Autodesk Inventor part; units mm, degrees
ref_plane "YZ Plane" through (0, 0, 0) normal (1, 0, 0) x (0, 1, 0)
ref_plane "XZ Plane" through (0, 0, 0) normal (0, 1, 0) x (-1, 0, 0)
ref_plane "XY Plane" through (0, 0, 0) normal (0, 0, 1) x (1, 0, 0)
sketch "Sketch1" plane through (0, 0, 0) normal (0, 0, 1) x (1, 0, 0)
  line L0 (-30, 30) -> (30, 30)
  line L1 (30, 30) -> (30, -30)
  line L2 (30, -30) -> (-30, -30)
  line L3 (-30, -30) -> (-30, 30)
  point P0 (0, 0)
  dimension "d0" = 60
  dimension "d1" = 60
  dimension "d2" = 30
  dimension "d3" = 30
extrude "Extrusion1" add sketch "Sketch1" along normal blind 10
sketch "Sketch2" plane through (0, 0, 10) normal (0, 0, 1) x (1, 0, 0)
  line L0 (30, 30) -> (-30, 30)
  line L1 (30, -30) -> (30, 30)
  line L2 (-30, 30) -> (30, 30)
  line L3 (30, 30) -> (30, -5)
  line L4 (30, -5) -> (-30, -5)
  line L5 (-30, -5) -> (-30, 30)
  point P0 (0, 0)
  dimension "d6" = 35
extrude "Extrusion2" add sketch "Sketch2" along normal blind 20
sketch "Sketch3" plane through (0, 0, 10) normal (0, 0, 1) x (1, 0, 0)
  line L0 (-30, -5) -> (30, -5)
  line L1 (-30, -30) -> (30, -30)
  line L2 (-30, -5) -> (30, -5)
  line L3 (30, -5) -> (30, -30)
  line L4 (30, -30) -> (-30, -30)
  line L5 (-30, -30) -> (-30, -5)
  point P0 (0, 0)
extrude "Extrusion3" add sketch "Sketch3" along normal blind 50
sketch "Sketch4" plane through (0, 0, 0) normal (0, 0, -1) x (-1, 0, 0)
  circle A0 centre (-20, 20) radius 1.95
  circle A1 centre (20, 20) radius 1.95
  circle A2 centre (20, 5) radius 1.95
  circle A3 centre (-20, 5) radius 1.95
  line L0 (-30, 30) -> (30, 30)
  line L1 (-30, -30) -> (-30, 30)
  line L2 (30, 30) -> (30, -30)
  point P0 (0, 0)
  dimension "d11" = 10
  dimension "d12" = 10
  dimension "d13" = 10
  dimension "d14" = 10
  dimension "d15" = 10
  dimension "d16" = 25
  dimension "d17" = 25
  dimension "d18" = 10
  dimension "d19" = 3.9
  dimension "d20" = 3.9
  dimension "d21" = 3.9
  dimension "d22" = 3.9
extrude "Extrusion4" cut sketch "Sketch4" against normal blind 30
sketch "Sketch5" plane through (0, 0, 0) normal (0, 0, -1) x (-1, 0, 0)
  circle A0 centre (-20, 20) radius 1.95
  circle A1 centre (-20, 20) radius 4.5
  circle A2 centre (-20, 5) radius 1.95
  circle A3 centre (-20, 5) radius 4.5
  circle A4 centre (20, 20) radius 1.95
  circle A5 centre (20, 20) radius 4.5
  circle A6 centre (20, 5) radius 1.95
  circle A7 centre (20, 5) radius 4.5
  point P0 (0, 0)
  dimension "d25" = 9
  dimension "d26" = 9
  dimension "d27" = 9
  dimension "d28" = 9
extrude "Extrusion5" cut sketch "Sketch5" against normal blind 20
sketch "Sketch6" plane through (-30, -30, 0) normal (-1, 0, 0) x (0, 0, 1)
  circle A0 centre (15, 10) radius 1.95
  circle A1 centre (45, 10) radius 1.95
  line L0 (0, 60) -> (0, 0)
  line L1 (0, 0) -> (60, 0)
  line L2 (60, 25) -> (60, 0)
  point P0 (0, 30)
  dimension "d31" = 15
  dimension "d32" = 10
  dimension "d33" = 15
  dimension "d34" = 10
  dimension "d35" = 3.9
  dimension "d36" = 3.9
extrude "Extrusion6" cut sketch "Sketch6" against normal blind 15
sketch "Sketch7" plane through (30, -30, 0) normal (1, 0, 0) x (0, 0, -1)
  circle A0 centre (-45, 10) radius 1.95
  circle A1 centre (-45, 10) radius 1.95
  circle A2 centre (-15, 10) radius 1.95
  circle A3 centre (-15, 10) radius 1.95
  point P0 (0, 30)
extrude "Extrusion7" cut sketch "Sketch7" against normal blind 15
sketch "Sketch8" plane through (0, 0, 0) normal (0, 0, -1) x (-1, 0, 0)
  circle A0 centre (0, -20) radius 1.95
  line L0 (30, -30) -> (-30, -30)
  line L1 (-30, -30) -> (-30, 30)
  point P0 (0, 0)
  dimension "d41" = 10
  dimension "d42" = 30
  dimension "d43" = 3.9
extrude "Extrusion8" cut sketch "Sketch8" against normal blind 15
sketch "Sketch9" plane through (0, 0, 60) normal (0, 0, 1) x (1, 0, 0)
  circle A0 centre (0, -20) radius 1.95
  circle A1 centre (0, -20) radius 1.95
  point P0 (0, 0)
extrude "Extrusion9" cut sketch "Sketch9" against normal blind 15
properties part number "Base_V2b"
Geometry: final body of the model. Coordinates: model frame, mm. A direction names the side the tool comes from. Round coordinates to 2 decimals unless told otherwise and drop trailing zeros. Order: outer loops, then holes, each group sorted by start corner. A loop starts at its lowest first (then second) coordinate and runs counter-clockwise, first axis right, second up. Notation, with made-up numbers: (12.25, 27.5) -> (50.25, 27.5) arc R27 ccw to (50.25, 50.5) -> close; hole circle Ø6 at (88, 11). An arc over 180 degrees is marked (long way). Put each result on its own line as item: value. Start each with the question number.
Q1. Line query: probe 1 along Y at (x, z) = (20, 22); probe 2 along Y at (x, z) = (20, 12.5); probe 3 along X at (y, z) = (7, 16). Output: solid intervals per line, ascending.
Q2. Reachability of faces 1 (the flat face through (-15, -20, 45)), 2 (the cylindrical face through (-0.9, -21.73, 7.4)), 3 (the flat face through (15, -20, 15)) from +Z, -Z, +X, -X, +Y, -Y: full face, straight path, thin tool, end or side. Return the list, or none.
Q3. Section A-A on x = 20. Return the cut outline in (y, z).
Q4. First-contact query: pin 1 (11.5 mm diameter, centred on x = -20, y = 5, fed in from +Z); pin 2 (8 mm diameter, centred on x = 20, y = 5, fed in from -Z); pin 3 (1.2 mm diameter, centred on x = 0.5, y = -21, fed in from +Z). Flat tips, straight axial feed; report the tip coordinate or a pass-through.
Q5. Pull-direction query (X, two-part tool) for faces 4 (the flat face through (0, -20, 45)), 5 (the flat face through (30, -6, 23)), 6 (the cylindrical face through (-22.605, -21.187, 13.453)); classes: +X half, -X half, draft (parallel to the pull), parting line (faces both ways), or undercut.
Q6. Section B-B on y = 20. Return the cut outline in (x, z).
Q7. Section C-C on y = -20. Return the cut outline in (x, z), and give its area (3 significant figures).
Q8. Section D-D on x = 0. Return the cut outline in (y, z).
Ans:
1. probe 1: y = -30 to 3.05, 6.95 to 18.05, 21.95 to 30
1. probe 2: y = -30 to 0.5, 9.5 to 15.5, 24.5 to 30
1. probe 3: x = -30 to -24.03, -15.97 to 15.97, 24.03 to 30
2. face 1: -X
2. face 2: -Z
2. face 3: +X
3. outline: (-30, 0) -> (0.5, 0) -> (0.5, 20) -> (3.05, 20) -> (3.05, 30) -> (-5, 30) -> (-5, 60) -> (-30, 60) -> close; (6.95, 20) -> (9.5, 20) -> (9.5, 0) -> (15.5, 0) -> (15.5, 20) -> (18.05, 20) -> (18.05, 30) -> (6.95, 30) -> close; (21.95, 20) -> (24.5, 20) -> (24.5, 0) -> (30, 0) -> (30, 30) -> (21.95, 30) -> close; hole circle Ø3.9 at (-20, 15); hole circle Ø3.9 at (-20, 45)
4. pin 1: stops at z = 30
4. pin 2: stops at z = 20
4. pin 3: stops at z = 45
5. face 4: undercut
5. face 5: +X half
5. face 6: draft
6. outline: (-30, 0) -> (-24.5, 0) -> (-24.5, 20) -> (-21.95, 20) -> (-21.95, 30) -> (-30, 30) -> close; (-18.05, 20) -> (-15.5, 20) -> (-15.5, 0) -> (15.5, 0) -> (15.5, 20) -> (18.05, 20) -> (18.05, 30) -> (-18.05, 30) -> close; (21.95, 20) -> (24.5, 20) -> (24.5, 0) -> (30, 0) -> (30, 30) -> (21.95, 30) -> close
7. outline: (-30, 0) -> (-1.95, 0) -> (-1.95, 15) -> (1.95, 15) -> (1.95, 0) -> (30, 0) -> (30, 13.05) -> (15, 13.05) -> (15, 16.95) -> (30, 16.95) -> (30, 43.05) -> (15, 43.05) -> (15, 46.95) -> (30, 46.95) -> (30, 60) -> (1.95, 60) -> (1.95, 45) -> (-1.95, 45) -> (-1.95, 60) -> (-30, 60) -> (-30, 46.95) -> (-15, 46.95) -> (-15, 43.05) -> (-30, 43.05) -> (-30, 16.95) -> (-15, 16.95) -> (-15, 13.05) -> (-30, 13.05) -> close
7. area: 3,250 mm2
8. outline: (-30, 0) -> (-21.95, 0) -> (-21.95, 15) -> (-18.05, 15) -> (-18.05, 0) -> (30, 0) -> (30, 30) -> (-5, 30) -> (-5, 60) -> (-18.05, 60) -> (-18.05, 45) -> (-21.95, 45) -> (-21.95, 60) -> (-30, 60) -> close
